```python
from build123d import *

# Parameters (mm, degrees)
F0_W     = 1270
F0_H     = 1651
F1_DEPTH = 304.8
F2_W     = 304.8
F2_H     = 762
F3_DEPTH = 635
F5_DEPTH = 304.8
F6_R     = 317.5
F7_DEPTH = 304.8


with BuildPart() as f1:
    # F0 (on Top) → F1 (new body)
    with BuildSketch(Plane.XY):
        with Locations((601.1569073796, 821.8028554339)):
            Rectangle(F0_W, F0_H)
    extrude(amount=F1_DEPTH)

    # F2 (on face) → F3 (join)
    with BuildSketch(Plane.XY.offset(304.8)):
        with Locations((1083.7569073796, 1266.3028554339)):
            Rectangle(F2_W, F2_H)
    extrude(amount=F3_DEPTH)

    # F4 (on face) → F5 (join)
    with BuildSketch(Plane.XY.offset(304.8)):
        with BuildLine():
            ThreePointArc((-33.8430926204, -3.6971445661), (601.1569073796, -638.6971445661), (1236.1569073796, -3.6971445661))
            Line((1236.1569073796, -3.6971445661), (-33.8430926204, -3.6971445661))
        make_face()
    extrude(amount=-F5_DEPTH)

    # F6 (on face) → F7 (cut)
    with BuildSketch(Plane.XY.offset(304.8)):
        with Locations((601.1569073796, -3.6971445661)):
            Circle(F6_R)
    extrude(amount=-F7_DEPTH, mode=Mode.SUBTRACT)


solid = f1.part
```
Design review of the part built by this model. Coordinates are the model's own, in mm. A direction names the side the tool comes from. Round coordinates to 2 decimals unless told otherwise and drop trailing zeros. Order: outer loops, then holes, each group sorted by start corner. A loop starts at its lowest first (then second) coordinate and runs counter-clockwise, first axis right, second up. Notation, with made-up numbers: (10, 57) - (52, 57) arc R29 cw to (52, 93) - close; hole circle Ø11 at (25.5, 33). An arc over 180 degrees is marked (long way). Return JSON: item names as keys, results as strings.
Q1. Consider section C-C on x = 851. Write out the cut boundary in (y, z), plus the area to 3 significant figures.
Computed values:
{"outline": "(-587.48, 0) - (-199.62, 0) - (-199.62, 304.8) - (-587.48, 304.8) - close; (192.22, 0) - (1647.3, 0) - (1647.3, 304.8) - (192.22, 304.8) - close", "area": "562,000 mm2"}
Q2. Consider section D-D on y = 1411.5. Write out the cut boundary in (x, z), plus the area to 3 significant figures.
Computed values:
{"outline": "(-33.84, 0) - (1236.16, 0) - (1236.16, 939.8) - (931.36, 939.8) - (931.36, 304.8) - (-33.84, 304.8) - close", "area": "581,000 mm2"}
Q3. Consider section A-A on y = -136.5. Write out the cut boundary in (x, z).
Computed values:
{"outline": "(-19.8, 0) - (312.77, 0) - (312.77, 304.8) - (-19.8, 304.8) - close; (889.55, 0) - (1222.11, 0) - (1222.11, 304.8) - (889.55, 304.8) - close"}
Q4. For pin 1 Ø10 at (x, y) = (1010, 36.5) entering from -Z; pin 2 Ø1 at (x, y) = (812.5, 697) entering from +Z; pin 3 Ø3 at (y, z) = (945, 448.5) entering from -X, all flat-tipped, find the tip position at first contact; note any pin that passes through.
Computed values:
{"pin 1": "stops at z = 0", "pin 2": "stops at z = 304.8", "pin 3": "stops at x = 931.36"}
Q5. Consider section B-B on z = 167.5. Write out the cut boundary in (x, y), plus the area to 3 significant figures.
Computed values:
{"outline": "(-33.84, -3.7) arc R635 ccw to (1236.16, -3.7) - (1236.16, 1647.3) - (-33.84, 1647.3) - close; hole circle Ø635 at (601.16, -3.7)", "area": "2,410,000 mm2"}
Q6. The part is to be moulded in two halves that separate along X. For faces 1 (the cylindrical face through (894.446, -125.302, 154.534)), 2 (the cylindrical face through (587.194, -638.544, 154.534)), 3 (the flat face through (931.357, 1261, 618)), 4 (the flat face through (1082, 1272, 939.8)), say which applies: pulls with the +X half, pulls with the -X half, needs draft (parallel to the pull), parting line crosses it, or undercut.
Computed values:
{"face 1": "undercut", "face 2": "parting line crosses it", "face 3": "pulls with the -X half", "face 4": "needs draft"}
Q7. Machinability: for faces 5 (the flat face through (1236.157, 994, 359)), 6 (the flat face through (1082, 885.303, 618)), which of the approach directions +Z, -Z, +X, -X, +Y, -Y give a long, thin tool a straight path to every point of the face, cutting with its end or side? Answer none if there is none.
Computed values:
{"face 5": "+Z, -Z, +X, +Y, -Y", "face 6": "+Z, +X, -X, -Y"}
Q8. Wall thickness on L1, parallel to Y at x = 1055.5, z = 434.5; L2, parallel to Z at x = 682, y = 1391.5; L3, parallel to X at y = 1232, z = 898.5: over which ranges is each line inside the solid? List them lowest first. Write a range as [from, to].
Computed values:
{"L1": "y = [885.3, 1647.3]", "L2": "z = [0, 304.8]", "L3": "x = [931.36, 1236.16]"}
